```python
from build123d import *

# Parameters (mm, degrees)
SKETCH1_W           = 180
SKETCH1_H           = 90
BOSS_EXTRUDE1_DEPTH = 22
SKETCH2_W           = 23
SKETCH2_H           = 90
CUT_EXTRUDE1_DEPTH  = 6
BOSS_EXTRUDE2_REACH = 116.562
SKETCH4_R           = 17.5
SKETCH4_R_2         = 7.5
BOSS_EXTRUDE3_DEPTH = 10
SKETCH5_R           = 7.5
CUT_EXTRUDE2_DEPTH  = 115.561578352
SKETCH6_W           = 90
SKETCH6_H           = 125
BOSS_EXTRUDE4_DEPTH = 22
CUT_EXTRUDE3_DEPTH  = 245.0397404
SKETCH9_R           = 22.5
BOSS_EXTRUDE5_DEPTH = 20
BOSS_EXTRUDE6_START = -12
SKETCH9_3_R         = 22.5
SKETCH9_3_R_2       = 11
BOSS_EXTRUDE6_DEPTH = 8
CUT_EXTRUDE4_DEPTH  = 5


with BuildPart() as part:
    # Sketch1 → Boss-Extrude1 (new body)
    with BuildSketch(Plane(origin=(0, 0, 0), x_dir=(1, 0, 0), z_dir=(0, 1, 0))):
        Rectangle(SKETCH1_W, SKETCH1_H)
    extrude(amount=BOSS_EXTRUDE1_DEPTH)

    # Sketch2 → Cut-Extrude1 (cut)
    with BuildSketch(Plane(origin=(0, 22, 0), x_dir=(1, 0, 0), z_dir=(0, 1, 0))):
        with Locations((-36.5, 0)):
            Rectangle(SKETCH2_W, SKETCH2_H)
    extrude(amount=-CUT_EXTRUDE1_DEPTH, mode=Mode.SUBTRACT)

    # Boss-Extrude2: up to this face of the body (flat: up to its plane)
    boss_extrude2_end = Plane(part.part.faces().sort_by_distance((32.5, 22, 0))[0])
    # Sketch3 → Boss-Extrude2 (add, up to the picked face)
    with BuildSketch(Plane(origin=(0, 35.306663677, 16.463767656), x_dir=(1, 0, 0), z_dir=(0, 0.9063077870366496, 0.4226182617407003)), mode=Mode.PRIVATE) as boss_extrude2_sk1:
        with BuildLine():
            Line((4, -31.486248658), (4, 8.513751342))
            ThreePointArc((4, 8.513751342), (32, 36.513751342), (60, 8.513751342))
            Line((60, 8.513751342), (60, -31.486248658))
            Line((60, -31.486248658), (4, -31.486248658))
        make_face()
    boss_extrude2_tool1 = split(extrude(boss_extrude2_sk1.sketch, amount=-BOSS_EXTRUDE2_REACH, mode=Mode.PRIVATE), bisect_by=boss_extrude2_end, keep=Keep.BOTH, mode=Mode.PRIVATE)
    add(boss_extrude2_tool1.solids().sort_by(Axis((32, 35.232426, 16.622971), (0, -0.9063077870366496, -0.4226182617407003)))[0])

    # Sketch4 → Boss-Extrude3 (add)
    with BuildSketch(Plane(origin=(0, 44.369741547, 20.689950274), x_dir=(1, 0, 0), z_dir=(0, 0.9063077870366496, 0.4226182617407003))):
        with Locations(Location((32, 8.513751342, 0), (0, 0, 270))):
            Circle(SKETCH4_R)
        with Locations(Location((32, 8.513751342, 0), (0, 0, 270))):
            Circle(SKETCH4_R_2, mode=Mode.SUBTRACT)
    extrude(amount=-BOSS_EXTRUDE3_DEPTH)

    # Sketch5 → Cut-Extrude2 (cut, through all)
    with BuildSketch(Plane(origin=(0, 35.306663677, 16.463767656), x_dir=(1, 0, 0), z_dir=(0, 0.9063077870366496, 0.42261826174070033))):
        with Locations(Location((32, 8.513751342, 0), (0, 0, 270))):
            Circle(SKETCH5_R)
    extrude(amount=-CUT_EXTRUDE2_DEPTH, mode=Mode.SUBTRACT)

    # Sketch6 → Boss-Extrude4 (add)
    with BuildSketch(Plane(origin=(-60.39090645, -42.286167935, 0), x_dir=(0, 0, 1), z_dir=(-0.8191520442889891, -0.5735764363510502, 0))):
        with Locations((0, 114.121879272)):
            Rectangle(SKETCH6_W, SKETCH6_H)
    extrude(amount=-BOSS_EXTRUDE4_DEPTH)

    # Sketch8 → Cut-Extrude3 (cut, through all)
    with BuildSketch(Plane(origin=(-101.306148094, 144.680173471, 0), x_dir=(0.8191520442889889, 0.5735764363510504, 0), z_dir=(-0.5735764363510503, 0.8191520442889889, 0))):
        Polygon((-73.723683986, 18.662115607), (-68.723683986, 15.775364262), (-68.723683986, -18.451133047), (-73.723683986, -21.337884393), align=None)
    extrude(amount=-CUT_EXTRUDE3_DEPTH, mode=Mode.SUBTRACT)

    # Sketch9 → Boss-Extrude5 (add)
    with BuildSketch(Plane(origin=(-101.306148094, 144.680173471, 0), x_dir=(0, 0, -1), z_dir=(-0.5735764363510415, 0.819152044288995, 0))):
        with BuildLine():
            ThreePointArc((45, 18.723683986), (0, -26.276316014), (-45, 18.723683986))
            Line((-45, 18.723683986), (-45, 73.723683986))
            Line((-45, 73.723683986), (-21.337884393, 73.723683986))
            Line((-21.337884393, 73.723683986), (-18.451133047, 68.723683986))
            Line((-18.451133047, 68.723683986), (15.775364262, 68.723683986))
            Line((15.775364262, 68.723683986), (18.662115607, 73.723683986))
            Line((18.662115607, 73.723683986), (45, 73.723683986))
            Line((45, 73.723683986), (45, 18.723683986))
        make_face()
        with Locations(Location((0, 18.723683986, 0), (0, 0, 90))):
            Circle(SKETCH9_R, mode=Mode.SUBTRACT)
    extrude(amount=-BOSS_EXTRUDE5_DEPTH)

    # Sketch9<3> → Boss-Extrude6 (add)
    with BuildSketch(Plane(origin=(-101.306148094, 144.680173471, 0), x_dir=(0, 0, -1), z_dir=(-0.5735764363510415, 0.819152044288995, 0)).offset(BOSS_EXTRUDE6_START)):
        with Locations(Location((0, 18.723683986, 0), (0, 0, 90))):
            Circle(SKETCH9_3_R)
        with Locations(Location((0, 18.723683986, 0), (0, 0, 90))):
            Circle(SKETCH9_3_R_2, mode=Mode.SUBTRACT)
    extrude(amount=-BOSS_EXTRUDE6_DEPTH)

    # Sketch11 → Cut-Extrude4 (cut)
    with BuildSketch(Plane(origin=(-101.306148094, 144.680173471, 0), x_dir=(0.8191520442889889, 0.5735764363510504, 0), z_dir=(-0.5735764363510503, 0.8191520442889889, 0))):
        with BuildLine():
            Line((-36.33759894, 14), (-68.723683986, 14))
            Line((-68.723683986, 14), (-68.723683986, 0))
            Line((-68.723683986, 0), (-41.223683986, 0))
            ThreePointArc((-41.223683986, 0), (-39.96707221, 7.414071538), (-36.33759894, 14))
        make_face()
        with BuildLine():
            Line((-41.223683986, 0), (-68.723683986, 0))
            Line((-68.723683986, 0), (-68.723683986, -14))
            Line((-68.723683986, -14), (-36.33759894, -14))
            ThreePointArc((-36.33759894, -14), (-39.96707221, -7.414071538), (-41.223683986, 0))
        make_face()
        with BuildLine():
            Line((24.043125575, 14), (-1.109769032, 14))
            ThreePointArc((-1.109769032, 14), (2.519704238, 7.414071538), (3.776316014, 0))
            ThreePointArc((3.776316014, 0), (2.519704238, -7.414071538), (-1.109769032, -14))
            Line((-1.109769032, -14), (24.043125575, -14))
            ThreePointArc((24.043125575, -14), (26.276316014, 0), (24.043125575, 14))
        make_face()
    extrude(amount=-CUT_EXTRUDE4_DEPTH, mode=Mode.SUBTRACT)


solid = part.part
```
Build history of the part. All positions in model axes, mm. A direction names the side the tool comes from. Give positions to 0.01 mm unless a question says otherwise; leave off trailing zeros. Loops run counter-clockwise (first coordinate to the right, second up) from the corner with the lowest first, then second, coordinate; pieces in that order, holes last.
1) Band-saw the part on D-D on z = -36.5. List the corners of the cut face in (x, y).
Values follow:
outline: (-161.7, 102.39) - (-90, 0) - (90, 0) - (90, 22) - (-25, 22) - (-25, 16) - (-48, 16) - (-48, 22) - (-78.55, 22) - (-132.2, 98.63) - (-83.61, 132.65) - (-95.08, 149.04) - close
2) Probe line 1 along X through (y, z) = (51.5, 3); line 2 along Y through (x, z) = (-20, -6); line 3 along X through (y, z) = (33, 19.5). List the from-to ranges inside material, lowest first.
Values follow:
line 1: x = -119.96 to -99.2, 18.02 to 45.98
line 2: y = 0 to 22
line 3: x = -109.22 to -86.25, 4 to 60
3) Drop flat-ended pins along their axis: P1, Ø13.5, axis at y = 29, z = 14.5, coming from the -X side; P2, Ø20.5, axis at x = -92, y = 147, coming from the -Z side; P3, Ø3, axis at x = -94, z = -7, coming from the +Y side. Give the stop position or say it passes through.
Values follow:
P1: stops at x = -110.88
P2: stops at z = -41.49
P3: stops at y = 144.74
4) Two-plate mould, pull along X, no slides. Class faces 5 (the face through (-126.35, 51.91, -32.02)), 6 (the face through (32.33, 25.859, -5.603)), 7 (the face through (-1, 0, -1)), 8 (the face through (31.38, 39.76, -21.74)): released by +X, released by -X, zero draft, split by the parting line, or undercut.
Values follow:
face 5: released by -X
face 6: undercut
face 7: zero draft
face 8: undercut
5) Band-saw the part on B-B on x = -27.5. List the corners of the cut face in (y, z).
Values follow:
outline: (0, -45) - (16, -45) - (16, 45) - (0, 45) - close
6) Band-saw the part on A-A on y = 28.5. State how many separate pieces and enclosed holes the cut face has, then the cut area to 3 significant figures.
Values follow:
separate pieces: 2
enclosed holes: 1
area: 4,880 mm2
7) Band-saw the part on C-C on y = 76. List the corners of the cut face in (x, z).
Values follow:
outline: (-143.22, -45) - (-116.36, -45) - (-116.36, 45) - (-143.22, 45) - (-143.22, 21.34) - (-137.11, 18.45) - (-137.11, -15.78) - (-143.22, -18.66) - close
8) 3-axis set-ups, long thin cutter, end or side, ignore diameter. For faces 1 (the face through (-88.29, 147.69, -0.2)), 2 (the face through (-121.265, 53.368, 1.098)), 3 (the face through (-101.31, 130.03, -4.68)), 4 (the face through (4, 30, 17)): which of +Z, -Z, +X, -X, +Y, -Y reach the whole face in a straight line?
Values follow:
face 1: -X, +Y
face 2: -X, -Y
face 3: none
face 4: +Z, -Z, +Y
